The figure shows three views and two pictorial views of one solid part (mm, origin at its lowest corner). Answer the questions. Give positions to 0.01 mm unless a question says otherwise; leave off trailing zeros. Loops run counter-clockwise (first coordinate to the right, second up) from the corner with the lowest first, then second, coordinate; pieces in that order, holes last. Notation, with made-up numbers: (-34.75, 53) - (3.25, 53) arc R25 ccw to (3.25, 82) - close; hole circle Ø11 at (5, 57.25). An arc over 180 degrees is marked (long way). Use a Markdown table: item, result. Add a question column.
Item 1: A cutting plane is placed at B-B (x = 6). Determine the outline of the cut face in (y, z).
Item 2: Each of these flat-tipped pins is pushed along its axis until it touches: P1, Ø5, axis at x = 5.5, z = 50.5, coming from the +Y side; P2, Ø3, axis at x = 38.5, y = 3.5, coming from the +Z side; P3, Ø1.8, axis at x = 86.5, z = 52.5, coming from the +Y side; P4, Ø2, axis at x = 12.5, y = 4.5, coming from the +Z side. Where does it stop, or does it pass through?
Item 3: A cutting plane is placed at C-C (x = 30.5). Determine the outline of the cut face in (y, z), plus the area to 4 significant figures.
Item 4: A cutting plane is placed at A-A (y = 1.65). Determine the outline of the cut face in (x, z).
Item 5: Consider probe 1 along X at (y, z) = (1.1, 6); probe 2 along Z at (x, y) = (87, 1.8); probe 3 along Z at (x, y) = (4.5, 3.2). Determine where each line is inside the solid, lowest interval first. Write a range as [from, to].
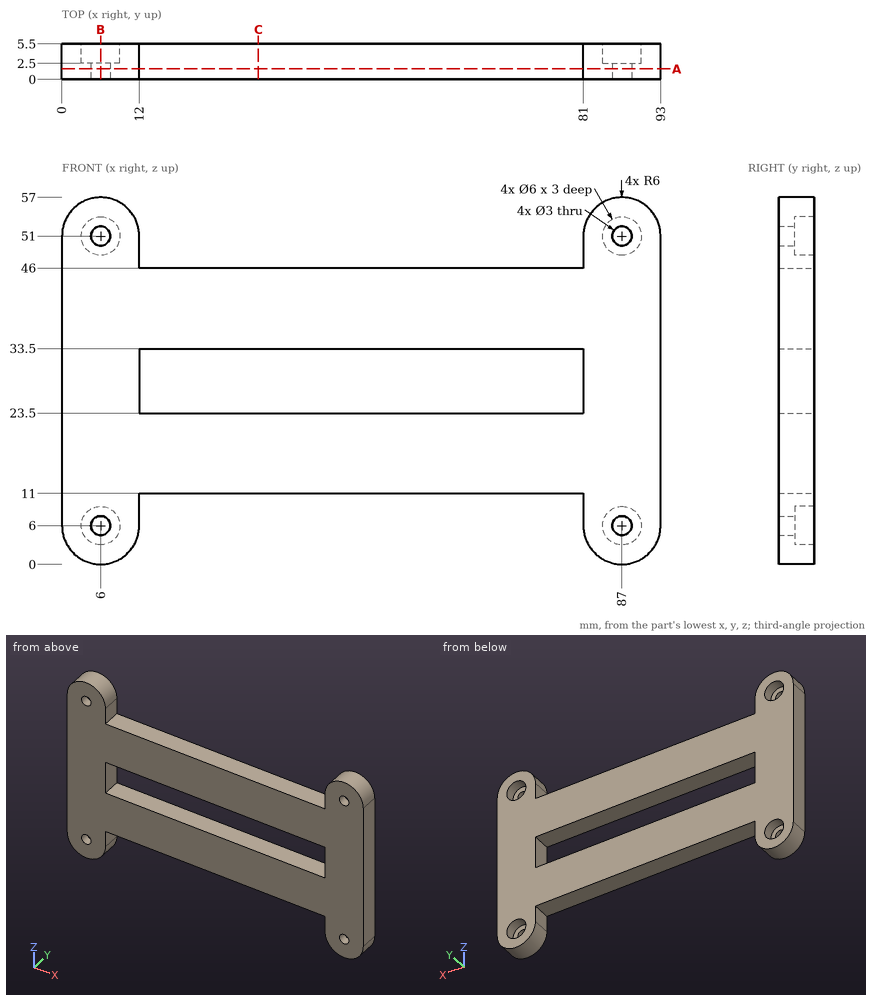
Geometry says:
| question | item | result |
|---|---|---|
| 1 | outline | (0, 0) - (5.5, 0) - (5.5, 3) - (2.5, 3) - (2.5, 4.5) - (0, 4.5) - close; (0, 7.5) - (2.5, 7.5) - (2.5, 9) - (5.5, 9) - (5.5, 48) - (2.5, 48) - (2.5, 49.5) - (0, 49.5) - close; (0, 52.5) - (2.5, 52.5) - (2.5, 54) - (5.5, 54) - (5.5, 57) - (0, 57) - close |
| 2 | P1 | y = 5.5 |
| 2 | P2 | z = 46 |
| 2 | P3 | y = 2.5 |
| 2 | P4 | z = 53.4 |
| 3 | outline | (0, 11) - (5.5, 11) - (5.5, 23.5) - (0, 23.5) - close; (0, 33.5) - (5.5, 33.5) - (5.5, 46) - (0, 46) - close |
| 3 | area | 137.5 mm² |
| 4 | outline | (0, 6) arc R6 ccw to (12, 6) - (12, 11) - (81, 11) - (81, 6) arc R6 ccw to (93, 6) - (93, 51) arc R6 ccw to (81, 51) - (81, 46) - (12, 46) - (12, 51) arc R6 ccw to (0, 51) - close; hole circle Ø3 at (6, 6); hole circle Ø3 at (6, 51); hole (12, 23.5) - (81, 23.5) - (81, 33.5) - (12, 33.5) - close; hole circle Ø3 at (87, 6); hole circle Ø3 at (87, 51) |
| 5 | probe 1 | [0, 4.5], [7.5, 12], [81, 85.5], [88.5, 93] |
| 5 | probe 2 | [0, 4.5], [7.5, 49.5], [52.5, 57] |
| 5 | probe 3 | [0.19, 3.4], [8.6, 48.4], [53.6, 56.81] |
